Check sheet for the modelled part. Datum: model origin and axes. Units: mm. Round coordinates to 2 decimals unless told otherwise and drop trailing zeros. Write each loop counter-clockwise with the first axis right and the second up, starting at its lowest first coordinate (ties: lowest second). Pieces come first, ordered by that corner, then holes.
Item 1: Cross-section at C-C on z = -28. Enter the section's corners in (x, y), plus the area to 3 significant figures.
Item 2: Material ranges on line 1 (Y direction, x = 7.5, z = -4); line 2 (Y direction, x = 5.5, z = -7); line 3 (Z direction, x = 5.75, y = -13.5), recorded low to high.
Item 3: Cross-section at D-D on y = -8. Enter the section's corners in (x, z), plus the area to 3 significant figures.
Item 4: Cross-section at B-B on x = 2.25. Enter the section's corners in (y, z), plus the area to 3 significant figures.
Item 5: Cross-section at A-A on z = -15.5. Enter the section's corners in (x, y).
Item 6: Go/stop test with flat-tipped pins: pin 1 Ø2 at (x, z) = (2.5, -29.5) entering from +Y; pin 2 Ø12 at (y, z) = (-2.5, -35.5) entering from +X; pin 3 Ø1 at (x, y) = (7, 21) entering from +Z; pin 4 Ø1 at (x, y) = (7, -7.5) entering from +Z. Record where each tip stops, or that it passes through.
from build123d import *

# Parameters (mm, degrees)
F1_DEPTH = 10
F2_R     = 3


with BuildPart() as f1:
    # F0 (on Right) → F1 (new body)
    with BuildSketch(Plane.YZ):
        with BuildLine():
            ThreePointArc((0, -40.5), (-28.653264, -28.622377), (-40.499976, 0.043681))
            Line((-40.499976, 0.043681), (-43.792324, 0.043681))
            Line((-43.792324, 0.043681), (-50, -41.5))
            Line((-50, -41.5), (0, -41.5))
            Line((0, -41.5), (0, -40.5))
        make_face()
        with BuildLine():
            ThreePointArc((40.499976, 0.043681), (28.653264, -28.622377), (0, -40.5))
            Line((0, -40.5), (0, -41.5))
            Line((0, -41.5), (50, -41.5))
            Line((50, -41.5), (43.792324, 0.043681))
            Line((43.792324, 0.043681), (40.499976, 0.043681))
        make_face()
    extrude(amount=F1_DEPTH)

    # F2
    f2_edges = [f1.edges().sort_by_distance(p)[0] for p in [
        (5, -43.792324, 0.043681),
        (5, 43.792324, 0.043681),
    ]]
    fillet(f2_edges, radius=F2_R)


solid = f1.part
Response values:
1. outline: (0, -47.98) - (10, -47.98) - (10, -29.26) - (0, -29.26) - close; (0, 29.26) - (10, 29.26) - (10, 47.98) - (0, 47.98) - close
1. area: 374 mm2
2. line 1: y = -44.4 to -40.3, 40.3 to 44.4
2. line 2: y = -44.84 to -39.89, 39.89 to 44.84
2. line 3: z = -41.5 to -38.18
3. outline: (0, -41.5) - (10, -41.5) - (10, -39.7) - (0, -39.7) - close
3. area: 18.0 mm2
4. outline: (-50, -41.5) - (50, -41.5) - (44.17, -2.51) arc R3 ccw to (41.21, 0.04) - (40.5, 0.04) arc R40.5 cw to (-40.5, 0.04) - (-41.21, 0.04) arc R3 ccw to (-44.17, -2.51) - close
4. area: 1,310 mm2
5. outline: (0, -46.11) - (10, -46.11) - (10, -37.42) - (0, -37.42) - close; (0, 37.42) - (10, 37.42) - (10, 46.11) - (0, 46.11) - close
6. pin 1: stops at y = 48.36
6. pin 2: stops at x = 10
6. pin 3: stops at z = -34.32
6. pin 4: stops at z = -39.7
